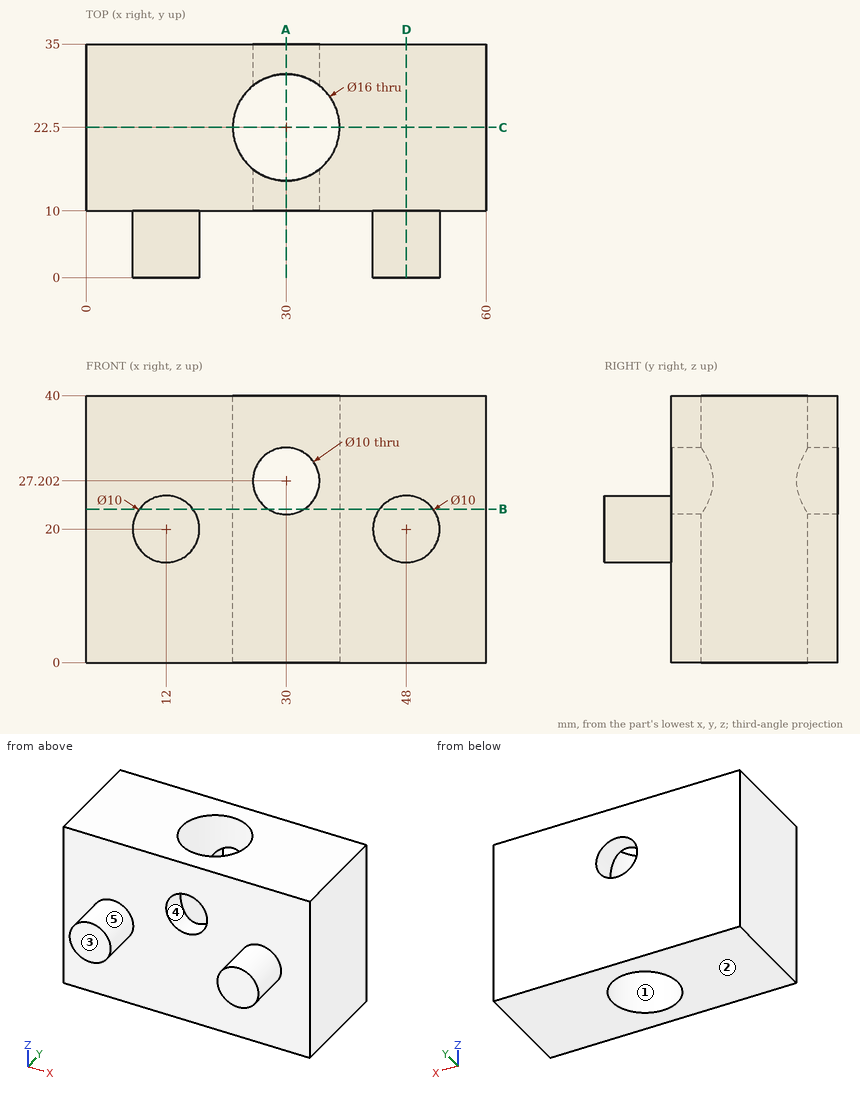
The drawing under review shows one solid part. Ordinate dimensions are in mm from its lowest x, y, z. A direction names the side the tool comes from. Round coordinates to 2 decimals unless told otherwise and drop trailing zeros. Write each loop counter-clockwise with the first axis right and the second up, starting at its lowest first coordinate (ties: lowest second). Pieces come first, ordered by that corner, then holes. Notation, with made-up numbers: (82.25, -39) -> (101.25, -39) arc R12 cw to (101.25, -30) -> close; hole circle Ø2 at (18, 85.25). An arc over 180 degrees is marked (long way). One line per question, with ' | ' between items.
(1) Wall thickness on line 1 (Z direction, x = 30, y = 32); line 2 (Y direction, x = 30, z = 10); line 3 (Y direction, x = 35, z = 9.5) (1 decimal): over which ranges is each line inside the solid? List them lowest first. Write a range as [from, to].
Result sheet:
line 1: [0, 22.2], [32.2, 40] | line 2: [10, 14.5], [30.5, 35] | line 3: [10, 16.3], [28.7, 35]
(2) Insertion check: P1, Ø9, axis at x = 30, z = 27.2, coming from the +Y side; P2, Ø2, axis at x = 53.5, z = 7.5, coming from the -Y side. Each pin has a flat end and moves straight along its axis. Give the tip position at first contact, or say it passes through.
Result sheet:
P1: through | P2: y = 10
(3) Take a section at B-B, the plane z = 23. State the section outline as (x, y) points.
Result sheet:
outline: (0, 10) -> (8, 10) -> (8, 0) -> (16, 0) -> (16, 10) -> (27.29, 10) -> (27.29, 14.97) arc R8 cw to (27.29, 30.03) -> (27.29, 35) -> (0, 35) -> close; (32.71, 10) -> (44, 10) -> (44, 0) -> (52, 0) -> (52, 10) -> (60, 10) -> (60, 35) -> (32.71, 35) -> (32.71, 30.03) arc R8 cw to (32.71, 14.97) -> close
(4) Take a section at A-A, the plane x = 30. State the section outline as (y, z) points.
Result sheet:
outline: (10, 0) -> (14.5, 0) -> (14.5, 22.2) -> (10, 22.2) -> close; (10, 32.2) -> (14.5, 32.2) -> (14.5, 40) -> (10, 40) -> close; (30.5, 0) -> (35, 0) -> (35, 22.2) -> (30.5, 22.2) -> close; (30.5, 32.2) -> (35, 32.2) -> (35, 40) -> (30.5, 40) -> close
(5) Machinability: for the marked faces 4 and 5, which of the approach directions +Z, -Z, +X, -X, +Y, -Y give a long, thin tool a straight path to every point of the face, cutting with its end or side? Answer none if there is none.
Result sheet:
face 4: +Y, -Y | face 5: -Y
(6) Take a section at C-C, the plane y = 22.5. State the section outline as (x, z) points.
Result sheet:
outline: (0, 0) -> (22, 0) -> (22, 40) -> (0, 40) -> close; (38, 0) -> (60, 0) -> (60, 40) -> (38, 40) -> close
(7) Draft analysis for pull direction Y (two halves, no side actions). For the marked faces 1, 2 and 3, state which applies: released by +Y, released by -Y, zero draft, split by the parting line, or undercut.
Result sheet:
face 1: undercut | face 2: zero draft | face 3: released by -Y
(8) Take a section at D-D, the plane x = 48. State the section outline as (y, z) points, and give its area (3 significant figures).
Result sheet:
outline: (0, 15) -> (10, 15) -> (10, 0) -> (35, 0) -> (35, 40) -> (10, 40) -> (10, 25) -> (0, 25) -> close | area: 1,100 mm2
